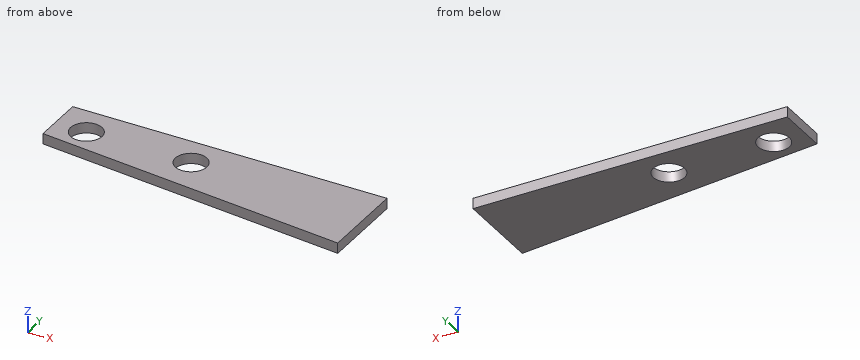
Autodesk Inventor part; units mm, degrees
ref_plane "YZ Plane" through (0, 0, 0) normal (1, 0, 0) x (0, 1, 0)
ref_plane "XZ Plane" through (0, 0, 0) normal (0, 1, 0) x (-1, 0, 0)
ref_plane "XY Plane" through (0, 0, 0) normal (0, 0, 1) x (1, 0, 0)
sketch "Sketch1" plane through (0, 0, 0) normal (0, 0, 1) x (1, 0, 0)
  line L0 (60, 0) -> (60, -16.5934)
  line L1 (60, 0) -> (0, 0)
  line L2 (0, 0) -> (0, -10)
  line L3 (0, -10) -> (60, -16.5934)
  dimension "d43" = 10
  dimension "d44" = 60
  dimension "d51" = 6.271
extrude "Plate1" add sketch "Sketch1" along normal blind 2
sketch "Sketch6" plane through (0, 0, 0) normal (0, 0, 1) x (1, 0, 0)
  line L0 (0, -10) -> (60, -16.5934)
  line L1 (0, 0) -> (0, -10)
  line L2 (60, 0) -> (0, 0)
  line L3 (60, -16.5934) -> (60, 0)
  circle A0 centre (6, -6) radius 3
  circle A1 centre (26, -6) radius 3
  dimension "d45" = 6
  dimension "d46" = 6
  dimension "d47" = 6
  dimension "d48" = 20
sketch "Sketch2" plane through (0, 0, 0) normal (0, 0, -1) x (-1, 0, 0)
  line L0 (-179.9406, -4.4713) -> (20.0594, -4.4713) construction
  line L1 (20.0594, -4.4713) -> (20.0594, -24.4713) construction
  line L2 (20.0594, -24.4713) -> (-179.9406, -24.4713) construction
  line L3 (-179.9406, -24.4713) -> (-179.9406, -4.4713) construction
  point P0 (0, 0)
  point P1 (-251, -525)
  dimension "d6" = 200
  dimension "d9" = 20
mark "Mark1"
extrude "Extrusion1" cut sketch "Sketch6" along normal through all contours A0 | A1
equation "\"d2\" = Thickness"
equation "\"BendReliefWidth\" = Thickness"
equation "\"BendReliefDepth\" = 0.5 * Thickness"
equation "\"CornerReliefSize\" = 4 * Thickness"
equation "\"MinimumRemnant\" = 2 * Thickness"
equation "\"TransitionRadius\" = BendRadius"
equation "\"JacobiRadiusSize\" = BendRadius"
equation "\"GapSize\" = Thickness"
properties part number "TRM 030 star conrtforce plate" material "AISI 304"
The listing builds one solid part. Answer for the finished solid, in the listing's coordinates (mm). Round coordinates to 2 decimals unless told otherwise and drop trailing zeros. Loops run counter-clockwise (first coordinate to the right, second up) from the corner with the lowest first, then second, coordinate; pieces in that order, holes last. Notation, with made-up numbers: (85.25, 1.25) -> (91.25, 1.25) arc R15 ccw to (91.25, 18.25) -> close; hole circle Ø11 at (14.5, 82.5). An arc over 180 degrees is marked (long way). Use one line per item in the form item = value.
1. The part is cut by section A-A on y = -6. Determine the outline of the cut face in (x, z), and give its area (3 significant figures).
Answer key:
outline = (0, 0) -> (3, 0) -> (3, 2) -> (0, 2) -> close; (9, 0) -> (23, 0) -> (23, 2) -> (9, 2) -> close; (29, 0) -> (60, 0) -> (60, 2) -> (29, 2) -> close
area = 96.0 mm²
2. The part is cut by section C-C on z = 0.9. Determine the outline of the cut face in (x, y).
Answer key:
outline = (0, -10) -> (60, -16.59) -> (60, 0) -> (0, 0) -> close; hole circle Ø6 at (6, -6); hole circle Ø6 at (26, -6)
3. The part is cut by section D-D on x = 6. Determine the outline of the cut face in (y, z), and give its area (3 significant figures).
Answer key:
outline = (-10.66, 0) -> (-9, 0) -> (-9, 2) -> (-10.66, 2) -> close; (-3, 0) -> (0, 0) -> (0, 2) -> (-3, 2) -> close
area = 9.32 mm²
4. Find the intervals of material crossed by probe 1 along X at (y, z) = (-6, 0.5); probe 2 along X at (y, z) = (-5, 1.85); probe 3 along Y at (x, z) = (26, 1.15), in increasing order. Write a range as [from, to].
Answer key:
probe_1 = [0, 3], [9, 23], [29, 60]
probe_2 = [0, 3.17], [8.83, 23.17], [28.83, 60]
probe_3 = [-12.86, -9], [-3, 0]
5. The part is cut by section B-B on x = 26. Determine the outline of the cut face in (y, z).
Answer key:
outline = (-12.86, 0) -> (-9, 0) -> (-9, 2) -> (-12.86, 2) -> close; (-3, 0) -> (0, 0) -> (0, 2) -> (-3, 2) -> close
